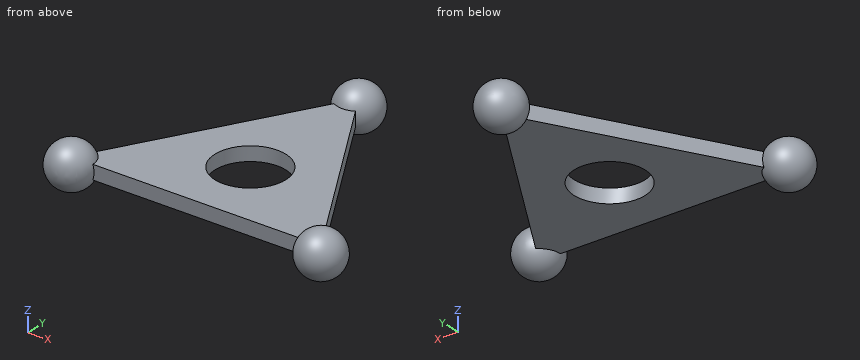
```python
from build123d import *

# Parameters (mm, degrees)
ESQUISSE1_R                  = 10
BOSS_EXTRU_1_DEPTH           = 2
R_P_TITION_CIRCULAIRE1_COUNT = 3


with BuildPart() as part:
    # Esquisse1 → Boss.-Extru.1 (new, symmetric)
    with BuildSketch(Plane.XY):
        Polygon((0, 40.414518843), (-35, -20.207259422), (35, -20.207259422), align=None)
        Circle(ESQUISSE1_R, mode=Mode.SUBTRACT)
    extrude(amount=BOSS_EXTRU_1_DEPTH, both=True)

    # Esquisse3 → Révolution1 (revolve)
    with BuildSketch(Plane.XY):
        with BuildLine():
            Line((0, 46.764518843), (0, 34.064518843))
            ThreePointArc((0, 34.064518843), (-6.35, 40.414518843), (0, 46.764518843))
        make_face()
    r_volution1 = revolve(axis=Axis((0, 46.764518843, 0), (0, -1, 0)))

    # Répétition circulaire1: Révolution1 ×3 about axis
    r_p_tition_circulaire1_axis = Axis((0, 0, 0), (0, 0, 1))
    for i in range(1, R_P_TITION_CIRCULAIRE1_COUNT):
        add(r_volution1.rotate(r_p_tition_circulaire1_axis, i * 360 / R_P_TITION_CIRCULAIRE1_COUNT))


solid = part.part
```
The listing builds one solid part. Answer for the finished solid, in the listing's coordinates (mm). Coordinates: 2 decimals unless noted, no trailing zeros. Write each loop counter-clockwise with the first axis right and the second up, starting at its lowest first coordinate (ties: lowest second). Pieces come first, ordered by that corner, then holes.
Q1. Section D-D, the plane y = 39 is taken. Write down the section's boundary in (x, z).
Returned:
outline: circle Ø12.38 at (0, 0)
Q2. Section C-C, the plane z = 4.25 is taken. Write down the section's boundary in (x, y).
Returned:
outline: circle Ø9.44 at (-35, -20.21); circle Ø9.44 at (0, 40.41); circle Ø9.44 at (35, -20.21)
Q3. Section A-A, the plane x = 0 is taken. Write down the section's boundary in (y, z).
Returned:
outline: (-20.21, -2) - (-10, -2) - (-10, 2) - (-20.21, 2) - close; (10, -2) - (34.39, -2) arc R6.35 ccw (long way) to (34.39, 2) - (10, 2) - close
Q4. Given P1, Ø6, axis at x = -13.5, z = 1.5, coming from the -Y side; P2, Ø2, axis at x = 24, y = -7, coming from the +Z side; P3, Ø4, axis at y = 37.5, z = -4, coming from the -X side, each flat-ended and moving along its own axis, determine where each tip first touches the part or whether it passes through.
Returned:
P1: stops at y = -20.21
P2: stops at z = 2
P3: stops at x = -5.62
Q5. Section B-B, the plane y = 0 is taken. Write down the section's boundary in (x, z).
Returned:
outline: (-23.33, -2) - (-10, -2) - (-10, 2) - (-23.33, 2) - close; (10, -2) - (23.33, -2) - (23.33, 2) - (10, 2) - close
Q6. Find the intervals of material crossed by line 1 along Z through (x, y) = (-11.5, 10); line 2 along Y through (x, z) = (0, 1.1); line 3 along X through (y, z) = (5.5, 1.5), in increasing order.
Returned:
line 1: z = -2 to 2
line 2: y = -20.21 to -10, 10 to 46.67
line 3: x = -20.16 to -8.35, 8.35 to 20.16
